```python
from build123d import *

# Parameters (mm, degrees)
SKETCH1_W           = 57.667844522
SKETCH1_H           = 30
BOSS_EXTRUDE1_DEPTH = 15
SKETCH2_R           = 4
CUT_EXTRUDE2_DEPTH  = 40
SKETCH3_R           = 8
CUT_EXTRUDE3_DEPTH  = 5
CUT_EXTRUDE5_DEPTH  = 16
SKETCH5_R           = 3
CUT_EXTRUDE6_DEPTH  = 5


with BuildPart() as part:
    # Sketch1 → Boss-Extrude1 (new body)
    with BuildSketch(Plane(origin=(0, 0, 0), x_dir=(1, 0, 0), z_dir=(0, 1, 0))):
        Rectangle(SKETCH1_W, SKETCH1_H)
    extrude(amount=BOSS_EXTRUDE1_DEPTH)

    # Sketch2 → Cut-Extrude2 (cut)
    with BuildSketch(Plane(origin=(0, 15, 0), x_dir=(1, 0, 0), z_dir=(0, 1, 0))):
        with Locations((0, 4)):
            Circle(SKETCH2_R)
    extrude(amount=-CUT_EXTRUDE2_DEPTH, mode=Mode.SUBTRACT)

    # Sketch3 → Cut-Extrude3 (cut)
    with BuildSketch(Plane(origin=(0, 15, 0), x_dir=(1, 0, 0), z_dir=(0, 1, 0))):
        with Locations((0, 4)):
            Circle(SKETCH3_R)
    extrude(amount=-CUT_EXTRUDE3_DEPTH, mode=Mode.SUBTRACT)

    # Sketch4 → Cut-Extrude5 (cut, through all)
    with BuildSketch(Plane(origin=(0, 15, 0), x_dir=(1, 0, 0), z_dir=(0, 1, 0))):
        with BuildLine():
            ThreePointArc((-11, 4), (-7.778174609, 11.778174577), (-4.5e-08, 15))
            Line((-4.5e-08, 15), (-28.833922261, 15))
            Line((-28.833922261, 15), (-28.833922261, -12))
            Line((-28.833922261, -12), (-11, -12))
            Line((-11, -12), (-11, 4))
        make_face()
        with BuildLine():
            ThreePointArc((-4.5e-08, 15), (7.778174577, 11.778174609), (11, 4))
            Line((11, 4), (11, -12))
            Line((11, -12), (28.833922261, -12))
            Line((28.833922261, -12), (28.833922261, 15))
            Line((28.833922261, 15), (-4.5e-08, 15))
        make_face()
        with BuildLine():
            Line((7.549834435, -12), (7.549834435, -4))
            ThreePointArc((7.549834435, -4), (0, -7), (-7.549834435, -4))
            Line((-7.549834435, -4), (-7.549834435, -12))
            Line((-7.549834435, -12), (7.549834435, -12))
        make_face()
    extrude(amount=-CUT_EXTRUDE5_DEPTH, mode=Mode.SUBTRACT)

    # Sketch5 → Cut-Extrude6 (cut)
    with BuildSketch(Plane(origin=(0, 0, 12), x_dir=(-1, 0, 0), z_dir=(0, 0, -1))):
        with Locations((21.333922261, 7.5)):
            Circle(SKETCH5_R)
        with Locations((-21.333922261, 7.5)):
            Circle(SKETCH5_R)
    extrude(amount=-CUT_EXTRUDE6_DEPTH, mode=Mode.SUBTRACT)


solid = part.part
```
Could you check a few things on this model? Use its own coordinates, in mm. A direction names the side the tool comes from. Round coordinates to 2 decimals unless told otherwise and drop trailing zeros. Write each loop counter-clockwise with the first axis right and the second up, starting at its lowest first coordinate (ties: lowest second). Pieces come first, ordered by that corner, then holes. Notation, with made-up numbers: M 14,70.25 L 41,70.25 A20 ccw 41,75.25 Z; hole C 75.25,89.5 d9. An arc over 180 degrees is marked long. Answer in a Markdown table with one row per item. Add a question column.
Q1. If we mould it in two halves opening along X, with no side actions, what happens to faces 5 (the flat face through (-7.55, 8, 8)), 6 (the flat face through (18, 8, 12)), 7 (the flat face through (-11, 8, 4))? For each: +X half, -X half, draft (parallel to the pull), parting line (faces both ways), or undercut.
Q2. Imagine slicing it at A-A (y = 7.5). Please give me the cut outline in (x, z), then the cut area to 3 significant figures.
Q3. Imagine slicing it at C-C (y = 11.5). Please give me the cut outline in (x, z).
Q4. On a 3-axis mill with a long thin cutter (end or side, diameter ignored), from which of +Z, -Z, +X, -X, +Y, -Y can I reach the whole of each face in a straight line? I mean faces 1 (the flat face through (0, 8, 12)), 2 (the flat face through (-18, 8, 12)), 3 (the cylindrical face through (-1.73, 12.54, 3.81)), 4 (the flat face through (11, 8, 4)). Say none if no direction works.
Q5. If I drill on line 1 (X direction, y = 2.5, z = -4); line 2 (Z direction, x = 5.5, y = 11.25); line 3 (Z direction, x = 0, y = 2.25), over which ranges is the centre line in solid material (lowest first)? Write a range as from..to.
Q6. Imagine slicing it at D-D (x = -19). Please give me the cut outline in (y, z), then the cut area to 3 significant figures.
Q7. Imagine slicing it at B-B (z = 10.5). Please give me the cut outline in (x, y).
Q8. Will these pins go through, and if not, where does the flat tip stop? pin 1 Ø3 at (x, y) = (-23, 12.5) entering from -Z; pin 2 Ø4.5 at (y, z) = (6.5, 7) entering from -X; pin 3 Ø2 at (y, z) = (5.5, -10) entering from +X.
Values:
| question | item | result |
|---|---|---|
| 1 | face 5 | undercut |
| 1 | face 6 | draft |
| 1 | face 7 | -X half |
| 2 | outline | M -28.83,12 L -24.33,12 L -24.33,15 L -28.83,15 Z; M -18.33,12 L -11,12 L -11,-4 A11 ccw 11,-4 L 11,12 L 18.33,12 L 18.33,15 L -18.33,15 Z; M 24.33,12 L 28.83,12 L 28.83,15 L 24.33,15 Z; hole M -7.55,4 A11 cw 7.55,4 L 7.55,12 L -7.55,12 Z; hole C 0,-4 d8 |
| 2 | area | 539 mm^2 |
| 3 | outline | M -28.83,12 L -11,12 L -11,-4 A11 ccw 11,-4 L 11,12 L 28.83,12 L 28.83,15 L -28.83,15 Z; hole C 0,-4 d16; hole M -7.55,4 A11 cw 7.55,4 L 7.55,12 L -7.55,12 Z |
| 4 | face 1 | +Y, -Y |
| 4 | face 2 | -Z, -X, +Y, -Y |
| 4 | face 3 | +Y |
| 4 | face 4 | -Z, +X, +Y, -Y |
| 5 | line 1 | -11..-4, 4..11 |
| 5 | line 2 | -13.53..-9.81, 1.81..5.53, 12..15 |
| 5 | line 3 | -15..-8, 0..7, 12..15 |
| 6 | outline | M 0,12 L 5.62,12 L 5.62,15 L 0,15 Z; M 9.38,12 L 15,12 L 15,15 L 9.38,15 Z |
| 6 | area | 33.7 mm^2 |
| 7 | outline | M -11,0 L -7.55,0 L -7.55,15 L -11,15 Z; M 7.55,0 L 11,0 L 11,15 L 7.55,15 Z |
| 8 | pin 1 | z = 12 |
| 8 | pin 2 | x = -11 |
| 8 | pin 3 | x = 9.8 |
